Here's the drawing with two shaded views (mm, measured from the low corner). I have some questions. A direction names the side the tool comes from. Coordinates: 2 decimals unless noted, no trailing zeros. Loops run counter-clockwise (first coordinate to the right, second up) from the corner with the lowest first, then second, coordinate; pieces in that order, holes last. Notation, with made-up numbers: (3.25, 52.5) -> (49.25, 52.5) arc R22 cw to (49.25, 67.5) -> close; hole circle Ø6 at (70.25, -38.75). An arc over 180 degrees is marked (long way). Answer as a JSON object with one key per item and string values. Group by question number.
1) I need wall thicknesses on probe 1 along Z at (x, y) = (17.75, 8.5) (1 decimal); probe 2 along X at (y, z) = (6.75, 35) (1 decimal); probe 3 along Y at (x, z) = (7, 5.5) (1 decimal). Which ranges of each line are inside material? Lowest first, please. Write a range as [from, to].
2) If we mould it in two halves opening along Y, with no side actions, what happens to the marked faces 1, 2 and 3? For each: +Y half, -Y half, draft (parallel to the pull), parting line (faces both ways), or undercut.
3) I want a section at B-B (z = 8). Write out the boundary of the cut face in (x, y) (1 decimal).
4) Which directions (+Z, -Z, +X, -X, +Y, -Y) give clear straight access to the entire face, cutting with the end or side of a thin tool? Please do the marked faces 4, 5 and 6.
5) I want a section at A-A (z = 19). Write out the boundary of the cut face in (x, y) (1 decimal).
6) I want a section at C-C (y = 1). Write out the boundary of the cut face in (x, z) (1 decimal).
7) I'm going to push flat-ended pins straight in: pin 1 (2 mm diameter, centred on y = 4, z = 6.5, fed in from -X); pin 2 (3 mm diameter, centred on x = 16, z = 19, fed in from -Y) (1 decimal); pin 3 (1 mm diameter, centred on y = 11.5, z = 15.5, fed in from -X). Where does each tip first touch, or does it pass through?
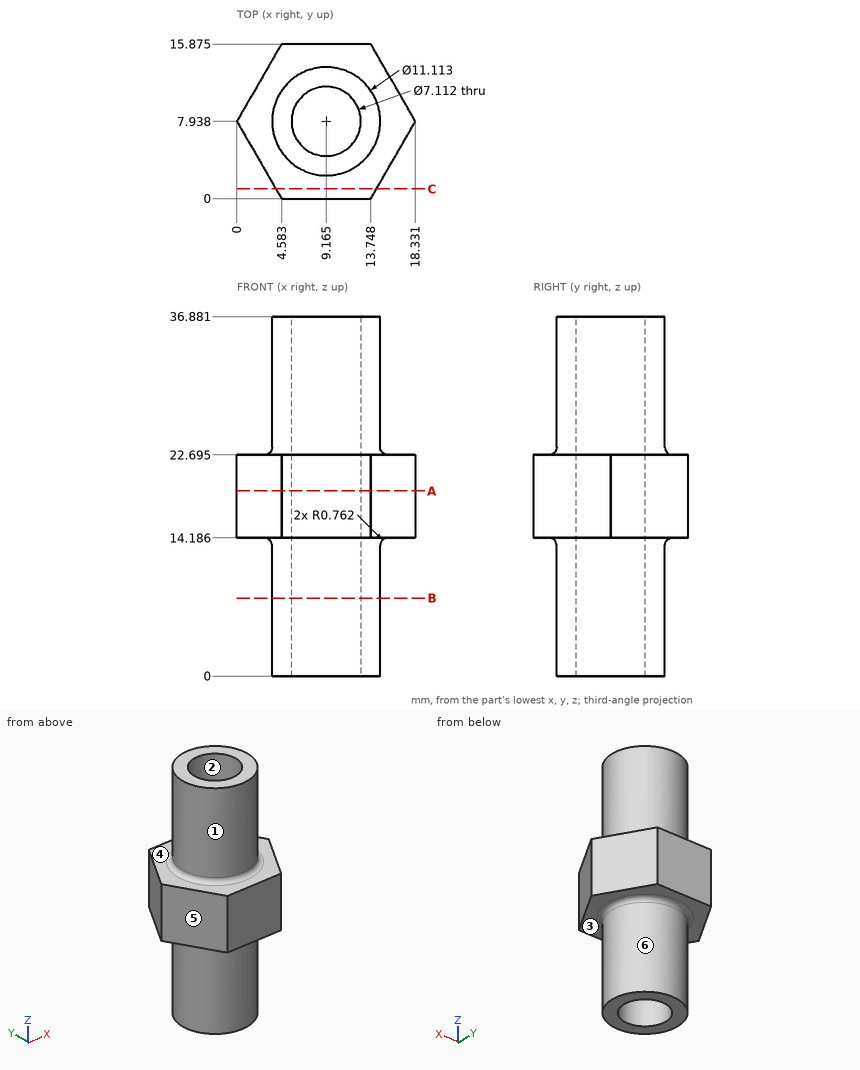
Determined:
{
 "1": {"probe 1": "[14.2, 22.7]", "probe 2": "[3.7, 5.8], [12.5, 14.6]", "probe 3": "[2.8, 5.1], [10.8, 13.1]"},
 "2": {"face 1": "parting line", "face 2": "undercut", "face 3": "draft"},
 "3": {"outline": "circle Ø11.1 at (9.2, 7.9); hole circle Ø7.1 at (9.2, 7.9)"},
 "4": {"face 4": "+Z", "face 5": "+Z, -Z, -X, -Y", "face 6": "-Z"},
 "5": {"outline": "(0, 7.9) -> (4.6, 0) -> (13.7, 0) -> (18.3, 7.9) -> (13.7, 15.9) -> (4.6, 15.9) -> close; hole circle Ø7.1 at (9.2, 7.9)"},
 "6": {"outline": "(4, 14.2) -> (14.3, 14.2) -> (14.3, 22.7) -> (4, 22.7) -> close"},
 "7": {"pin 1": "x = 4.45", "pin 2": "y = 1.3", "pin 3": "x = 1.77"}
}
